```python
from build123d import *

# Parameters (mm, degrees)
F0_R     = 12.45
F1_DEPTH = 12
F2_R     = 14.5
F3_DEPTH = 3
F4_R     = 9.95
F5_DEPTH = 70
F7_DEPTH = 20


with BuildPart() as f1:
    # F0 (on Front) → F1 (new body)
    with BuildSketch(Plane.XZ):
        Circle(F0_R)
    extrude(amount=F1_DEPTH)

    # F2 (on face) → F3 (join)
    with BuildSketch(Plane.XZ.offset(12)):
        Circle(F2_R)
    extrude(amount=F3_DEPTH)

    # F4 (on face) → F5 (join)
    with BuildSketch(Plane.XZ.offset(15)):
        Circle(F4_R)
    extrude(amount=F5_DEPTH)

    # F6 (on face) → F7 (join)
    with BuildSketch(Plane.XZ.offset(15)):
        with BuildLine():
            Line((2, 9.7469225913), (2, 12.3389626793))
            ThreePointArc((2, 12.3389626793), (0, 12.5), (-2, 12.3389626793))
            Line((-2, 12.3389626793), (-2, 9.7469225913))
            ThreePointArc((-2, 9.7469225913), (0, 9.95), (2, 9.7469225913))
        make_face()
        with BuildLine():
            ThreePointArc((-7.3471313431, 6.7098555146), (-5.8484632603, 8.049719094), (-4.1110633656, 9.0609965238))
            Line((-4.1110633656, 9.0609965238), (-5.6346263027, 11.1580010051))
            ThreePointArc((-5.6346263027, 11.1580010051), (-7.3473156537, 10.1127124297), (-8.8706942802, 8.8068599959))
            Line((-8.8706942802, 8.8068599959), (-7.3471313431, 6.7098555146))
        make_face()
        with BuildLine():
            ThreePointArc((-9.887908233, 1.109851691), (-9.4630123371, 3.074719094), (-8.6518402555, 4.9140777561))
            Line((-8.6518402555, 4.9140777561), (-11.1170168717, 5.7150621934))
            ThreePointArc((-11.1170168717, 5.7150621934), (-11.8882064537, 3.8627124297), (-12.3530848492, 1.9108361283))
            Line((-12.3530848492, 1.9108361283), (-9.887908233, 1.109851691))
        make_face()
        with BuildLine():
            ThreePointArc((-8.6518402555, -4.9140777561), (-9.4630123371, -3.074719094), (-9.887908233, -1.109851691))
            Line((-9.887908233, -1.109851691), (-12.3530848492, -1.9108361283))
            ThreePointArc((-12.3530848492, -1.9108361283), (-11.8882064537, -3.8627124297), (-11.1170168717, -5.7150621934))
            Line((-11.1170168717, -5.7150621934), (-8.6518402555, -4.9140777561))
        make_face()
        with BuildLine():
            ThreePointArc((-4.1110633656, -9.0609965238), (-5.8484632603, -8.049719094), (-7.3471313431, -6.7098555146))
            Line((-7.3471313431, -6.7098555146), (-8.8706942802, -8.8068599959))
            ThreePointArc((-8.8706942802, -8.8068599959), (-7.3473156537, -10.1127124297), (-5.6346263027, -11.1580010051))
            Line((-5.6346263027, -11.1580010051), (-4.1110633656, -9.0609965238))
        make_face()
        with BuildLine():
            ThreePointArc((2, -9.7469225913), (0, -9.95), (-2, -9.7469225913))
            Line((-2, -9.7469225913), (-2, -12.3389626793))
            ThreePointArc((-2, -12.3389626793), (0, -12.5), (2, -12.3389626793))
            Line((2, -12.3389626793), (2, -9.7469225913))
        make_face()
        with BuildLine():
            Line((8.8706942802, -8.8068599959), (7.3471313431, -6.7098555146))
            ThreePointArc((7.3471313431, -6.7098555146), (5.8484632603, -8.049719094), (4.1110633656, -9.0609965238))
            Line((4.1110633656, -9.0609965238), (5.6346263027, -11.1580010051))
            ThreePointArc((5.6346263027, -11.1580010051), (7.3473156537, -10.1127124297), (8.8706942802, -8.8068599959))
        make_face()
        with BuildLine():
            Line((12.3530848492, -1.9108361283), (9.887908233, -1.109851691))
            ThreePointArc((9.887908233, -1.109851691), (9.4630123371, -3.074719094), (8.6518402555, -4.9140777561))
            Line((8.6518402555, -4.9140777561), (11.1170168717, -5.7150621934))
            ThreePointArc((11.1170168717, -5.7150621934), (11.8882064537, -3.8627124297), (12.3530848492, -1.9108361283))
        make_face()
        with BuildLine():
            Line((11.1170168717, 5.7150621934), (8.6518402555, 4.9140777561))
            ThreePointArc((8.6518402555, 4.9140777561), (9.4630123371, 3.074719094), (9.887908233, 1.109851691))
            Line((9.887908233, 1.109851691), (12.3530848492, 1.9108361283))
            ThreePointArc((12.3530848492, 1.9108361283), (11.8882064537, 3.8627124297), (11.1170168717, 5.7150621934))
        make_face()
        with BuildLine():
            Line((5.6346263027, 11.1580010051), (4.1110633656, 9.0609965238))
            ThreePointArc((4.1110633656, 9.0609965238), (5.8484632603, 8.049719094), (7.3471313431, 6.7098555146))
            Line((7.3471313431, 6.7098555146), (8.8706942802, 8.8068599959))
            ThreePointArc((8.8706942802, 8.8068599959), (7.3473156537, 10.1127124297), (5.6346263027, 11.1580010051))
        make_face()
    extrude(amount=F7_DEPTH)


solid = f1.part
```
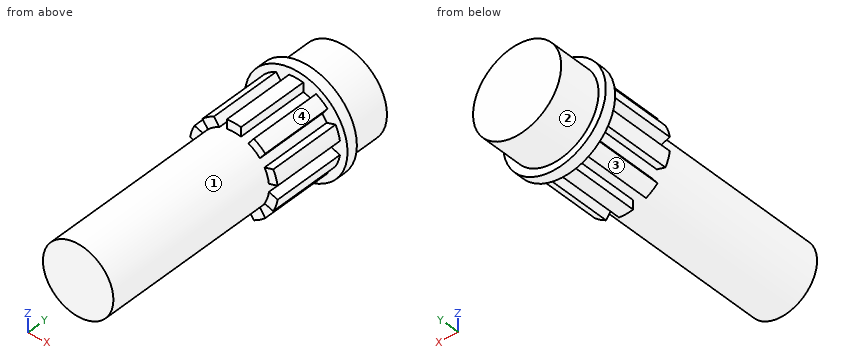
Geometry check sheet. Reference: the model listing, model coordinates, mm. Face numbers are marked on the shaded views. A direction names the side the tool comes from. Round coordinates to 2 decimals unless told otherwise and drop trailing zeros. Order: outer loops, then holes, each group sorted by start corner. A loop starts at its lowest first (then second) coordinate and runs counter-clockwise, first axis right, second up. Notation, with made-up numbers: M 1.5,-38 L 57.5,-38 A21 cw 57.5,-17 Z; hole C -7,53 d6. An arc over 180 degrees is marked long. Write item = value, one per line.
Q1. Set-up check for the marked faces 1, 2, 3 and 4: record each of +Z, -Z, +X, -X, +Y, -Y from which the full face is reachable in a straight line by a thin tool's end or side.
Answer block:
face_1 = -Y
face_2 = +Y
face_3 = -Z, -X, -Y
face_4 = +Z, +X, -Y
Q2. Section check D-D (z = 8). Enter the section's corners in (x, y), plus the area to 3 significant figures.
Answer block:
outline = M -12.09,-15 L -8.28,-15 L -8.28,-35 L -5.92,-35 L -5.92,-85 L 5.92,-85 L 5.92,-35 L 8.28,-35 L 8.28,-15 L 12.09,-15 L 12.09,-12 L 9.54,-12 L 9.54,0 L -9.54,0 L -9.54,-12 L -12.09,-12 Z
area = 1,220 mm^2
Q3. Scan lines: line 1 (Z direction, x = -0.25, y = -36.5); line 2 (Y direction, x = 10.5, z = -0.5); line 3 (Y direction, x = 3.75, z = 13). Record each from-to range of solid material in increasing order.
Answer block:
line_1 = -9.95 to 9.95
line_2 = -15 to 0
line_3 = -15 to -12
Q4. Section check A-A (z = 0). Enter the section's corners in (x, y).
Answer block:
outline = M -14.5,-15 L -9.95,-15 L -9.95,-85 L 9.95,-85 L 9.95,-15 L 14.5,-15 L 14.5,-12 L 12.45,-12 L 12.45,0 L -12.45,0 L -12.45,-12 L -14.5,-12 Z
Q5. Section check C-C (y = -54). Enter the section's corners in (x, z), plus the area to 3 significant figures.
Answer block:
outline = C 0,0 d19.9
area = 311 mm^2
Q6. Section check B-B (x = 0). Enter the section's corners in (y, z).
Answer block:
outline = M -85,-9.95 L -35,-9.95 L -35,-12.5 L -15,-12.5 L -15,-14.5 L -12,-14.5 L -12,-12.45 L 0,-12.45 L 0,12.45 L -12,12.45 L -12,14.5 L -15,14.5 L -15,12.5 L -35,12.5 L -35,9.95 L -85,9.95 Z
Q7. Depth check by flat-ended pin: pin 1 Ø2 at (y, z) = (-30, -11) entering from +X; pin 2 Ø0.8 at (y, z) = (-27, -11) entering from -X; pin 3 Ø3 at (y, z) = (-21, 11.5) entering from -X. Enter the tip coordinate at first touch or a pass-through.
Answer block:
pin_1 = 7.5
pin_2 = -6.62
pin_3 = -7.5
